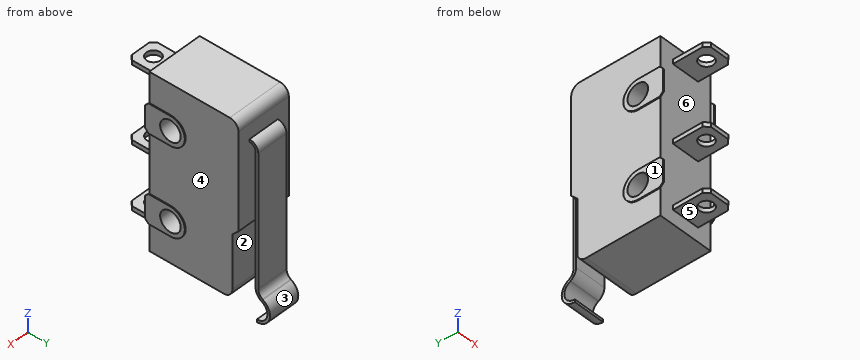
from build123d import *

# Parameters (mm, degrees)
EXTRUDE_1_DEPTH        = 3.2
SKETCH_3_W             = 0.5
SKETCH_3_H             = 3.9
EXTRUDE_3_DEPTH        = 1.6
CHAMFER_1_SIZE         = 0.5
SKETCH_4_R             = 0.8
CUT_EXTRUDE_1_DEPTH    = 22.107344693
EXTRUDE_4_DEPTH        = 0.1
PATTERN_LINEAR_1_COUNT = 2
PATTERN_LINEAR_1_PITCH = 10
MIRROR_1_COPY_1_DEPTH  = 0.1
SKETCH_6_R             = 1.175
CUT_EXTRUDE_2_DEPTH    = 24.230152819
EXTRUDE_2_DEPTH        = 1.8


with BuildPart() as part:
    # ｽｹｯﾁ1 → ﾎﾞｽ - 押し出し1 (new, symmetric)
    with BuildSketch(Plane(origin=(0, 0, 0), x_dir=(0, 0, -1), z_dir=(1, 0, 0))):
        with BuildLine():
            Line((12, 10.2), (12.7, 9.5))
            Line((12.7, 9.5), (18.8, 9.5))
            ThreePointArc((18.8, 9.5), (19.507106781, 9.207106781), (19.8, 8.5))
            Line((19.8, 8.5), (19.8, 0))
            Line((19.8, 0), (0, 0))
            Line((0, 0), (0, 9.2))
            ThreePointArc((0, 9.2), (0.292893219, 9.907106781), (1, 10.2))
            Line((1, 10.2), (12, 10.2))
        make_face()
    extrude(amount=EXTRUDE_1_DEPTH, both=True)

    # ｽｹｯﾁ3 → ﾎﾞｽ - 押し出し3 (add, symmetric)
    with BuildSketch(Plane(origin=(0, 0, 0), x_dir=(0, 0, -1), z_dir=(1, 0, 0))):
        with Locations((1.85, -1.95)):
            Rectangle(SKETCH_3_W, SKETCH_3_H)
        with Locations((10.65, -1.95)):
            Rectangle(SKETCH_3_W, SKETCH_3_H)
        with Locations((17.95, -1.95)):
            Rectangle(SKETCH_3_W, SKETCH_3_H)
    extrude(amount=EXTRUDE_3_DEPTH, both=True)

    # 面取り1
    chamfer_1_edges = [part.edges().sort_by_distance(p)[0] for p in [
        (-1.6, -3.9, -1.85),
        (1.6, -3.9, -1.85),
        (-1.6, -3.9, -10.65),
        (1.6, -3.9, -10.65),
        (-1.6, -3.9, -17.95),
        (1.6, -3.9, -17.95),
    ]]
    chamfer(chamfer_1_edges, length=CHAMFER_1_SIZE)

    # ｽｹｯﾁ4 → ｶｯﾄ - 押し出し1 (cut, through all)
    with BuildSketch(Plane(origin=(0, 0, -18.2), x_dir=(-1, 0, 0), z_dir=(0, 0, -1))):
        with Locations((0, -2.4)):
            Circle(SKETCH_4_R)
    extrude(amount=-CUT_EXTRUDE_1_DEPTH, mode=Mode.SUBTRACT)

    # ｽｹｯﾁ5 → ﾎﾞｽ - 押し出し4 (add)
    with BuildSketch(Plane(origin=(3.2, 0, 0), x_dir=(0, 0, -1), z_dir=(1, 0, 0))):
        with BuildLine():
            Line((3.45, 2.5), (3.45, 0))
            Line((3.45, 0), (3.85, -0.4))
            Line((3.85, -0.4), (6.35, -0.4))
            Line((6.35, -0.4), (6.75, 0))
            Line((6.75, 0), (6.75, 2.5))
            ThreePointArc((6.75, 2.5), (5.1, 4.15), (3.45, 2.5))
        make_face()
    extrude_4 = extrude(amount=EXTRUDE_4_DEPTH)

    # 直線ﾊﾟﾀｰﾝ1: ﾎﾞｽ - 押し出し4 ×2
    with Locations(*[(0, 0, -i * PATTERN_LINEAR_1_PITCH) for i in range(1, PATTERN_LINEAR_1_COUNT)]):
        add(extrude_4)

    # ﾐﾗｰ1: ﾎﾞｽ - 押し出し4 across plane
    add(extrude_4.mirror(Plane(origin=(0, 0, 0), x_dir=(0, 0, 1), z_dir=(1, 0, 0))))

    # ﾐﾗｰ1 copy 1 sketch → ﾐﾗｰ1 copy 1 (add)
    with BuildSketch(Plane(origin=(-3.2, 0, -10), x_dir=(0, 0, -1), z_dir=(-1, 0, 0))):
        with BuildLine():
            Line((3.45, -2.5), (3.45, 0))
            Line((3.45, 0), (3.85, 0.4))
            Line((3.85, 0.4), (6.35, 0.4))
            Line((6.35, 0.4), (6.75, 0))
            Line((6.75, 0), (6.75, -2.5))
            ThreePointArc((6.75, -2.5), (5.1, -4.15), (3.45, -2.5))
        make_face()
    extrude(amount=MIRROR_1_COPY_1_DEPTH)

    # ｽｹｯﾁ6 → ｶｯﾄ - 押し出し2 (cut, through all)
    with BuildSketch(Plane(origin=(3.3, 0, 0), x_dir=(0, 0, -1), z_dir=(1, 0, 0))):
        with Locations((5.1, 2.5)):
            Circle(SKETCH_6_R)
        with Locations((15.1, 2.5)):
            Circle(SKETCH_6_R)
    extrude(amount=-CUT_EXTRUDE_2_DEPTH, mode=Mode.SUBTRACT)

    # ｽｹｯﾁ2 → ﾎﾞｽ - 押し出し2 (add, symmetric)
    with BuildSketch(Plane(origin=(0, 0, 0), x_dir=(0, 0, -1), z_dir=(1, 0, 0))):
        with BuildLine():
            Line((3.683747293, 11.2), (18.683747293, 11.2))
            ThreePointArc((18.683747293, 11.2), (19.1692369, 11.325757561), (19.532618528, 11.671400315))
            Line((19.532618528, 11.671400315), (19.570248376, 11.737273482))
            ThreePointArc((19.570248376, 11.737273482), (21.257332173, 12.5), (22.4, 11.043183705))
            Line((22.4, 11.043183705), (22.1, 11.043183705))
            ThreePointArc((22.1, 11.043183705), (21.183255021, 12.209274007), (19.833722345, 11.59368526))
            Line((19.833722345, 11.59368526), (19.790473564, 11.517975834))
            ThreePointArc((19.790473564, 11.517975834), (19.317532977, 11.064960041), (18.683747293, 10.9))
            Line((18.683747293, 10.9), (3.683747293, 10.9))
            ThreePointArc((3.683747293, 10.9), (3.188772547, 10.694974747), (2.983747293, 10.2))
            Line((2.983747293, 10.2), (2.683747293, 10.2))
            ThreePointArc((2.683747293, 10.2), (2.976640512, 10.907106781), (3.683747293, 11.2))
        make_face()
    extrude(amount=EXTRUDE_2_DEPTH, both=True)


solid = part.part
CAD build for the part. Positions are in the model's coordinates, mm. Face numbers are marked on the shaded views. A direction names the side the tool comes from. Round coordinates to 2 decimals unless told otherwise and drop trailing zeros. Write each loop counter-clockwise with the first axis right and the second up, starting at its lowest first coordinate (ties: lowest second). Pieces come first, ordered by that corner, then holes. Notation, with made-up numbers: M 47.25,46.5 L 69.25,46.5 A21 cw 69.25,75.5 Z; hole C -6.75,31 d7. An arc over 180 degrees is marked long. Use a Markdown table: item, result. Add a question column.
1. Drill centre lines: probe 1 along Y at (x, z) = (1, -9.5); probe 2 along Y at (x, z) = (-1, -12.75); probe 3 along Z at (x, y) = (2.75, 2). Where is each one in solid material? Low to high.
2. Pull direction Y, two halves, no side cores. Call the marked faces 1, 2 and 3: released by +Y, released by -Y, zero draft, split by the parting line, or undercut.
3. Slice it at D-D on z = -15.1. Give the cut face in (x, y) (3 decimals), then the cut area to 3 significant figures.
4. Flat gauge pins, fed straight in: P1, Ø8, axis at y = 4.5, z = -13.5, coming from the -X side; P2, Ø2.5, axis at x = 0, y = -2.4, coming from the -Z side; P3, Ø1.6, axis at x = -0.5, y = -2.5, coming from the +Z side; P4, Ø1.5, axis at x = -1.5, z = -4.5, coming from the +Y side. Where does each tip first touch, or does it go through?
5. Slice it at A-A on z = -12.25. Give the cut face in (x, y), then the cut area to 3 significant figures.
6. 3-axis set-ups, long thin cutter, end or side, ignore diameter. For the marked faces 4, 5 and 6: which of +Z, -Z, +X, -X, +Y, -Y reach the whole face in a straight line?
7. Slice it at B-B on x = 0. Give the number of separate pieces and of enclosed holes in the cut face, then the cut area to 3 significant figures.
8. Slice it at C-C on y = -2.4. Give the cut face in (x, z), then the cut area to 3 significant figures.
Reply:
| question | item | result |
|---|---|---|
| 1 | probe 1 | y = 0 to 10.2, 10.9 to 11.2 |
| 1 | probe 2 | y = 0 to 9.5, 10.9 to 11.2 |
| 1 | probe 3 | z = -19.8 to -16.16, -14.04 to -6.16, -4.04 to 0 |
| 2 | face 1 | zero draft |
| 2 | face 2 | undercut |
| 2 | face 3 | released by +Y |
| 3 | outline | M -3.3,-0.4 L -3.2,-0.4 L -3.2,0 L 3.2,0 L 3.2,-0.4 L 3.3,-0.4 L 3.3,1.325 L -3.3,1.325 Z; M -3.3,3.675 L 3.3,3.675 L 3.3,4.15 L 3.2,4.15 L 3.2,9.5 L -3.2,9.5 L -3.2,4.15 L -3.3,4.15 Z; M -1.8,10.9 L 1.8,10.9 L 1.8,11.2 L -1.8,11.2 Z |
| 3 | area | 47.3 mm^2 |
| 4 | P1 | stops at x = -3.3 |
| 4 | P2 | stops at z = -18.2 |
| 4 | P3 | stops at z = -1.6 |
| 4 | P4 | stops at y = 11.2 |
| 5 | outline | M -3.2,0 L 3.2,0 L 3.2,9.95 L -3.2,9.95 Z; M -1.8,10.9 L 1.8,10.9 L 1.8,11.2 L -1.8,11.2 Z |
| 5 | area | 64.8 mm^2 |
| 6 | face 4 | +X, +Y |
| 6 | face 5 | -Z, +X, -X, -Y |
| 6 | face 6 | -Y |
| 7 | separate pieces | 4 |
| 7 | enclosed holes | 2 |
| 7 | area | 197 mm^2 |
| 8 | outline | M -1.6,-18.2 L -0.8,-18.2 L -0.8,-17.7 L -1.6,-17.7 Z; M -1.6,-10.9 L -0.8,-10.9 L -0.8,-10.4 L -1.6,-10.4 Z; M -1.6,-2.1 L -0.8,-2.1 L -0.8,-1.6 L -1.6,-1.6 Z; M 0.8,-18.2 L 1.6,-18.2 L 1.6,-17.7 L 0.8,-17.7 Z; M 0.8,-10.9 L 1.6,-10.9 L 1.6,-10.4 L 0.8,-10.4 Z; M 0.8,-2.1 L 1.6,-2.1 L 1.6,-1.6 L 0.8,-1.6 Z |
| 8 | area | 2.40 mm^2 |
